```python
from build123d import *

# Parameters (mm, degrees)
SKETCH1_W           = 4.25
SKETCH1_H           = 14
BOSS_EXTRUDE1_DEPTH = 2
SCALE1_SCALE        = 10
SKETCH2_R           = 3.05
CUT_EXTRUDE1_DEPTH  = 143.03321973
SKETCH4_R           = 3.1
CUT_EXTRUDE2_DEPTH  = 82.304166761


with BuildPart() as part:
    # Sketch1 → Boss-Extrude1 (new body)
    with BuildSketch(Plane(origin=(0, 0, 0), x_dir=(1, 0, 0), z_dir=(0, 1, 0))):
        with Locations((-0.020531401, -5.881038647)):
            Rectangle(SKETCH1_W, SKETCH1_H)
    extrude(amount=BOSS_EXTRUDE1_DEPTH)


with BuildPart() as part_1:
    # Scale1: scaled about (-0.020531401, 1, 5.881038647)
    add(part.part.scale(SCALE1_SCALE).moved(Location((0.184782609, -9, -52.929347823))))

    # Sketch2 → Cut-Extrude1 (cut, through all)
    with BuildSketch(Plane(origin=(0, 0, -64.118961353), x_dir=(-1, 0, 0), z_dir=(0, 0, -1))):
        with Locations((-13.229468599, 1)):
            Circle(SKETCH2_R)
    extrude(amount=-CUT_EXTRUDE1_DEPTH, mode=Mode.SUBTRACT)

    # Sketch4 → Cut-Extrude2 (cut, through all)
    with BuildSketch(Plane(origin=(0, 11, 0), x_dir=(1, 0, 0), z_dir=(0, 1, 0))):
        with Locations(Location((-0.020531401, 51.018961353, 0), (0, 0, 270))):
            Circle(SKETCH4_R)
    extrude(amount=-CUT_EXTRUDE2_DEPTH, mode=Mode.SUBTRACT)


solid = part_1.part
```
The listing builds one solid part. Answer for the finished solid, in the listing's coordinates (mm). Round coordinates to 2 decimals unless told otherwise and drop trailing zeros. Write each loop counter-clockwise with the first axis right and the second up, starting at its lowest first coordinate (ties: lowest second). Pieces come first, ordered by that corner, then holes. Notation, with made-up numbers: (16, 45) -> (32, 45) arc R36 cw to (32, 80) -> close; hole circle Ø5 at (-1.5, -17.5). An arc over 180 degrees is marked (long way). Use CSV: the item, a comma, the result in double quotes. Start each with the question number.
(1) Section C-C on z = 54 is taken. Give the vertices of the cut face in (x, y), then the cut area to 3 significant figures.
(2) The mould has two halves that part along X. Classify faces 1 (the face through (0.116, 1.14, -54.116)), 2 (the face through (0, 1, 75.881)), 3 (the face through (-21.271, 1, 7)): released by +X, released by -X, zero draft, split by the parting line, or undercut.
(3) Section A-A on z = -49.5 is taken. Give the vertices of the cut face in (x, y), then the cut area to 3 significant figures.
(4) Consider L1, parallel to X at y = -0.25, z = 35; L2, parallel to Y at x = 11, z = -47; L3, parallel to X at y = -1, z = 12. Determine where each line is inside the solid, lowest interval first. Write a range as from..to.
(5) Section B-B on y = 1 is taken. Give the vertices of the cut face in (x, z), then the cut area to 3 significant figures.
A:
1,outline,"(-21.27, -9) -> (21.23, -9) -> (21.23, 11) -> (-21.27, 11) -> close; hole circle Ø6.1 at (13.23, 1)"
1,area,"821 mm²"
2,face 1,"undercut"
2,face 2,"zero draft"
2,face 3,"released by -X"
3,outline,"(-21.27, -9) -> (-2.72, -9) -> (-2.72, 11) -> (-21.27, 11) -> close; (2.68, -9) -> (21.23, -9) -> (21.23, 11) -> (2.68, 11) -> close; hole circle Ø6.1 at (13.23, 1)"
3,area,"713 mm²"
4,L1,"x = -21.27..10.45, 16.01..21.23"
4,L2,"y = -9..-1.08, 3.08..11"
4,L3,"x = -21.27..10.93, 15.53..21.23"
5,outline,"(-21.27, -64.12) -> (10.18, -64.12) -> (10.18, 75.88) -> (-21.27, 75.88) -> close; (16.28, -64.12) -> (21.23, -64.12) -> (21.23, 75.88) -> (16.28, 75.88) -> close; hole circle Ø6.2 at (-0.02, -51.02)"
5,area,"5,070 mm²"
